Build history of the part. All positions in model axes, mm. A direction names the side the tool comes from. Give positions to 0.01 mm unless a question says otherwise; leave off trailing zeros. Loops run counter-clockwise (first coordinate to the right, second up) from the corner with the lowest first, then second, coordinate; pieces in that order, holes last.
1) Two-plate mould, pull along Y, no slides. Class faces 1 (the cylindrical face through (14.7, -50.4, 2)), 2 (the cylindrical face through (41.524, 33.614, 0.69)): +Y half, -Y half, draft (parallel to the pull), parting line (faces both ways), or undercut.
2) 3-axis set-ups, long thin cutter, end or side, ignore diameter. For faces 3 (the cylindrical face through (-14.91, -50.34, 1.97)), 4 (the cylindrical face through (-30.514, -29.87, 1.972)), 5 (the cylindrical face through (51.948, -7.596, 1.972)): which of +Z, -Z, +X, -X, +Y, -Y reach the whole face in a straight line?
3) Flat gauge pins, fed straight in: P1, Ø5, axis at x = -39.68, y = 34.38, coming from the +Z side; P2, Ø1.5, axis at y = 3, z = 1.5, coming from the -X side; P3, Ø1, axis at y = 25, z = 1, coming from the -X side. Where does each tip first touch, or does it go through?
4) Band-saw the part on A-A on y = -36.5. List the corners of the cut face in (x, z).
5) Band-saw the part on C-C on y = 17.5. List the corners of the cut face in (x, z).
6) Band-saw the part on B-B on x = -39. State how many separate pieces and enclosed holes the cut face has, then the cut area to 3 significant figures.
7) Wall check: line 1 (Y direction, x = -13, z = 0.95); line 2 (X direction, y = -46, z = 2.5); line 3 (X direction, y = 35, z = 1.5). Give the ranges that are in metal, low to high.
```python
from build123d import *

# Parameters (mm, degrees)
SKETCH_1_R               = 42.7
SKETCH_1_R_2             = 2
EXTRUDE_1_DEPTH          = 4
SKETCH_2_R               = 1
CUT_EXTRUDE_1_DEPTH      = 4
PATTERN_CIRCULAR_1_COUNT = 11


with BuildPart() as part:
    # 草图1 → 凸台-拉伸1 (new body)
    with BuildSketch(Plane.XY):
        with BuildLine():
            ThreePointArc((-57.90455435, 8.325418039), (-56.664135325, 3.740040393), (-52.478752132, 1.493510837))
            ThreePointArc((-52.478752132, 1.493510837), (-51.965625699, -7.471529009), (-49.932223308, -16.217986173))
            ThreePointArc((-49.932223308, -16.217986173), (-53.315148558, -19.552674205), (-53.213471728, -24.301778261))
            ThreePointArc((-53.213471728, -24.301778261), (-49.690922522, -27.488622249), (-44.95538855, -27.115734184))
            ThreePointArc((-44.95538855, -27.115734184), (-39.676852654, -34.380188532), (-33.237553958, -40.63883619))
            ThreePointArc((-33.237553958, -40.63883619), (-34.280583312, -45.27310175), (-31.627487821, -49.213331671))
            ThreePointArc((-31.627487821, -49.213331671), (-26.941192918, -49.989841552), (-23.159006743, -47.115925192))
            ThreePointArc((-23.159006743, -47.115925192), (-14.790959234, -50.373381115), (-5.990196072, -52.157142857))
            ThreePointArc((-5.990196072, -52.157142857), (-4.36217508, -56.619639374), (0, -58.5))
            ThreePointArc((0, -58.5), (4.36217508, -56.619639374), (5.990196072, -52.157142857))
            ThreePointArc((5.990196072, -52.157142857), (14.790959234, -50.373381115), (23.159006743, -47.115925192))
            ThreePointArc((23.159006743, -47.115925192), (26.941192918, -49.989841552), (31.627487821, -49.213331671))
            ThreePointArc((31.627487821, -49.213331671), (34.280583312, -45.27310175), (33.237553958, -40.63883619))
            ThreePointArc((33.237553958, -40.63883619), (39.676852654, -34.380188532), (44.95538855, -27.115734184))
            ThreePointArc((44.95538855, -27.115734184), (49.690922522, -27.488622249), (53.213471728, -24.301778261))
            ThreePointArc((53.213471728, -24.301778261), (53.315148558, -19.552674205), (49.932223308, -16.217986173))
            ThreePointArc((49.932223308, -16.217986173), (51.965625699, -7.471529009), (52.478752132, 1.493510837))
            ThreePointArc((52.478752132, 1.493510837), (56.664135325, 3.740040393), (57.90455435, 8.325418039))
            ThreePointArc((57.90455435, 8.325418039), (55.422530843, 12.375589248), (50.773764562, 13.351959864))
            ThreePointArc((50.773764562, 13.351959864), (47.755679756, 21.809288183), (43.34048271, 29.62857672))
            ThreePointArc((43.34048271, 29.62857672), (45.646885531, 33.781266636), (44.2113501, 38.309352936))
            ThreePointArc((44.2113501, 38.309352936), (39.933651182, 40.374690556), (35.494994318, 38.682752984))
            ThreePointArc((35.494994318, 38.682752984), (28.383642916, 44.165810474), (20.441916256, 48.35677884))
            ThreePointArc((20.441916256, 48.35677884), (20.137072107, 53.097179409), (16.481354575, 56.130338956))
            ThreePointArc((16.481354575, 56.130338956), (11.766119429, 55.555112887), (8.946814173, 51.732045351))
            ThreePointArc((8.946814173, 51.732045351), (0, 52.5), (-8.946814173, 51.732045351))
            ThreePointArc((-8.946814173, 51.732045351), (-11.766119429, 55.555112887), (-16.481354575, 56.130338956))
            ThreePointArc((-16.481354575, 56.130338956), (-20.137072107, 53.097179409), (-20.441916256, 48.35677884))
            ThreePointArc((-20.441916256, 48.35677884), (-28.383642916, 44.165810474), (-35.494994318, 38.682752984))
            ThreePointArc((-35.494994318, 38.682752984), (-39.933651182, 40.374690556), (-44.2113501, 38.309352936))
            ThreePointArc((-44.2113501, 38.309352936), (-45.646885531, 33.781266636), (-43.34048271, 29.62857672))
            ThreePointArc((-43.34048271, 29.62857672), (-47.755679756, 21.809288183), (-50.773764562, 13.351959864))
            ThreePointArc((-50.773764562, 13.351959864), (-55.422530843, 12.375589248), (-57.90455435, 8.325418039))
        make_face()
        Circle(SKETCH_1_R, mode=Mode.SUBTRACT)
        with Locations((-51.965625699, 7.471529009)):
            Circle(SKETCH_1_R_2, mode=Mode.SUBTRACT)
        with Locations((-39.676852654, 34.380188532)):
            Circle(SKETCH_1_R_2, mode=Mode.SUBTRACT)
        with Locations((-14.790959234, 50.373381115)):
            Circle(SKETCH_1_R_2, mode=Mode.SUBTRACT)
        with Locations((14.790959234, 50.373381115)):
            Circle(SKETCH_1_R_2, mode=Mode.SUBTRACT)
        with Locations((39.676852654, 34.380188532)):
            Circle(SKETCH_1_R_2, mode=Mode.SUBTRACT)
        with Locations((51.965625699, 7.471529009)):
            Circle(SKETCH_1_R_2, mode=Mode.SUBTRACT)
        with Locations((47.755679756, -21.809288183)):
            Circle(SKETCH_1_R_2, mode=Mode.SUBTRACT)
        with Locations((28.383642916, -44.165810474)):
            Circle(SKETCH_1_R_2, mode=Mode.SUBTRACT)
        with Locations((0, -52.5)):
            Circle(SKETCH_1_R_2, mode=Mode.SUBTRACT)
        with Locations((-28.383642916, -44.165810474)):
            Circle(SKETCH_1_R_2, mode=Mode.SUBTRACT)
        with Locations((-47.755679756, -21.809288183)):
            Circle(SKETCH_1_R_2, mode=Mode.SUBTRACT)
    extrude(amount=EXTRUDE_1_DEPTH)

    # 草图2 → 切除-拉伸1 (cut)
    with BuildSketch(Plane.XY.offset(4)):
        with Locations((0, -42.7)):
            Circle(SKETCH_2_R)
        with Locations((-42.7, 0)):
            Circle(SKETCH_2_R)
    extrude(amount=-CUT_EXTRUDE_1_DEPTH, mode=Mode.SUBTRACT)

    # 草图4 → 切除-旋转1 (revolve, cut)
    with BuildSketch(Plane(origin=(0, 0, 0), x_dir=(0, 0, -1), z_dir=(1, 0, 0)), mode=Mode.PRIVATE) as cut_revolve_1_sk:
        Polygon((-4, -52.5), (-4, -57.1), (-1.4, -54.5), (-1.4, -52.5), align=None)
    cut_revolve_1 = revolve(cut_revolve_1_sk.sketch.rotate(Axis((0, -52.5, 4), (0, 0, -1)), 270), axis=Axis((0, -52.5, 4), (0, 0, -1)), mode=Mode.SUBTRACT)

    # 阵列(圆周)1: 切除-旋转1 ×11 about axis
    pattern_circular_1_axis = Axis((0, 0, 0), (0, 0, 1))
    for i in range(1, PATTERN_CIRCULAR_1_COUNT):
        add(cut_revolve_1.rotate(pattern_circular_1_axis, i * 360 / PATTERN_CIRCULAR_1_COUNT), mode=Mode.SUBTRACT)


solid = part.part
```
Findings below:
1. face 1: -Y half
1. face 2: undercut
2. face 3: +Z, -Z, -Y
2. face 4: +Z, -Z
2. face 5: +Z, -Z, +X
3. P1: stops at z = 1.9
3. P2: stops at x = -56.67
3. P3: stops at x = -46.43
4. outline: (-37.74, 0) - (-22.16, 0) - (-22.16, 4) - (-37.74, 4) - close; (22.16, 0) - (37.74, 0) - (37.74, 4) - (22.16, 4) - close
5. outline: (-49.5, 0) - (-38.95, 0) - (-38.95, 4) - (-49.5, 4) - close; (38.95, 0) - (49.5, 0) - (49.5, 4) - (38.95, 4) - close
6. separate pieces: 3
6. enclosed holes: 0
6. area: 141 mm2
7. line 1: y = -50.87 to -40.67, 40.67 to 49.48, 51.26 to 56.1
7. line 2: x = -34.1 to -30.88, -25.88 to 25.88, 30.88 to 34.1
7. line 3: x = -45.64 to -41.68, -37.67 to -24.46, 24.46 to 37.67, 41.68 to 45.64
